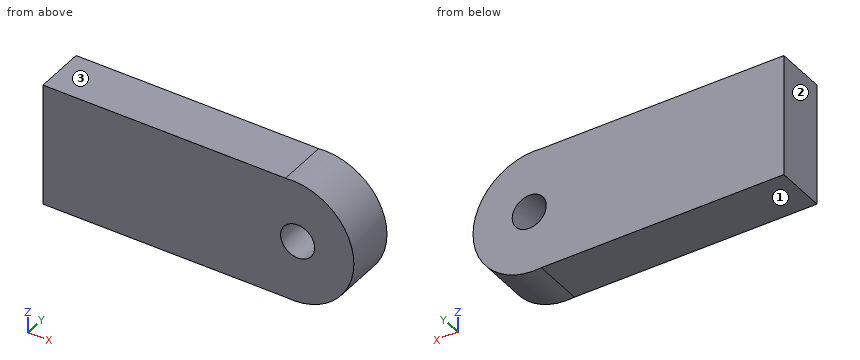
from build123d import *

# Parameters (mm, degrees)
F0_W     = 91.440002
F0_H     = 46.273064
F1_DEPTH = 19.05
F2_R     = 6.419279
F3_DEPTH = 70.358


with BuildPart() as f1:
    # F0 (on Front) → F1 (new body)
    with BuildSketch(Plane.XZ):
        with Locations((-15.024918, -0.368711)):
            Rectangle(F0_W, F0_H)
        with BuildLine():
            Line((30.695083, 22.767821), (30.695083, -23.505243))
            ThreePointArc((30.695083, -23.505243), (56.461966, -0.368711), (30.695083, 22.767821))
        make_face()
    extrude(amount=F1_DEPTH)

    # F2 (on face) → F3 (cut)
    with BuildSketch(Plane.XZ.offset(19.05)):
        with Locations((35.259977, 0)):
            Circle(F2_R)
    extrude(amount=-F3_DEPTH, mode=Mode.SUBTRACT)


solid = f1.part
Model file for the job. Use its own axes, mm. Face numbers are marked on the shaded views. A direction names the side the tool comes from. Round coordinates to 2 decimals unless told otherwise and drop trailing zeros. Order: outer loops, then holes, each group sorted by start corner. A loop starts at its lowest first (then second) coordinate and runs counter-clockwise, first axis right, second up.
(1) Band-saw the part on A-A (z = 0). List the corners of the cut face in (x, y).
(2) Band-saw the part on C-C (y = -16.5). List the corners of the cut face in (x, z), then the cut area to 3 significant figures.
(3) Drill centre lines: line 1 (Z direction, x = -51.5, y = -5); line 2 (X direction, y = -7.25, z = 0.5); line 3 (X direction, y = -16, z = 1.5). Where is each one in solid material? Low to high.
(4) Pin check, flat tips, straight feed: pin 1 (2 mm diameter, centred on x = 42, y = -17, fed in from +Z); pin 2 (2 mm diameter, centred on x = 5, y = -12.5, fed in from +Z); pin 3 (3 mm diameter, centred on x = 22.5, z = 13, fed in from +Y); pin 4 (9.5 mm diameter, centred on x = -3, y = -12, fed in from -Z). Stop position of each tip, or through.
(5) Band-saw the part on B-B (x = 35). List the corners of the cut face in (y, z), then the cut area to 3 significant figures.
(6) Band-saw the part on D-D (z = -13.5). List the corners of the cut face in (x, y), then the cut area to 3 significant figures.
(7) 3-axis set-ups, long thin cutter, end or side, ignore diameter. For the marked faces 1, 2 and 3: which of +Z, -Z, +X, -X, +Y, -Y reach the whole face in a straight line?
Verdict:
1. outline: (-60.74, -19.05) - (28.84, -19.05) - (28.84, 0) - (-60.74, 0) - close; (41.68, -19.05) - (56.46, -19.05) - (56.46, 0) - (41.68, 0) - close
2. outline: (-60.74, -23.51) - (30.7, -23.51) arc R23.27 ccw (long way) to (30.7, 22.77) - (-60.74, 22.77) - close; hole circle Ø12.84 at (35.26, 0)
2. area: 5,070 mm2
3. line 1: z = -23.51 to 22.77
3. line 2: x = -60.74 to 28.86, 41.66 to 56.45
3. line 3: x = -60.74 to 29.02, 41.5 to 56.39
4. pin 1: stops at z = 21.55
4. pin 2: stops at z = 22.77
4. pin 3: stops at y = 0
4. pin 4: stops at z = -23.51
5. outline: (-19.05, -23.57) - (0, -23.57) - (0, -6.41) - (-19.05, -6.41) - close; (-19.05, 6.41) - (0, 6.41) - (0, 22.83) - (-19.05, 22.83) - close
5. area: 640 mm2
6. outline: (-60.74, -19.05) - (52.4, -19.05) - (52.4, 0) - (-60.74, 0) - close
6. area: 2,160 mm2
7. face 1: -Z, -X, +Y, -Y
7. face 2: +Z, -Z, -X, +Y, -Y
7. face 3: +Z, -X, +Y, -Y
